Autodesk Inventor part; units mm, degrees
ref_plane "YZ Plane" through (0, 0, 0) normal (1, 0, 0) x (0, 1, 0)
ref_plane "XZ Plane" through (0, 0, 0) normal (0, 1, 0) x (-1, 0, 0)
ref_plane "XY Plane" through (0, 0, 0) normal (0, 0, 1) x (1, 0, 0)
sketch "Sketch1" plane through (0, 0, 0) normal (0, 0, 1) x (1, 0, 0)
  line L0 (-12.5, 71.5) -> (12.5, 71.5)
  line L1 (12.5, 71.5) -> (12.5, 0)
  line L2 (12.5, 0) -> (-12.5, 0)
  line L3 (-12.5, 0) -> (-12.5, 71.5)
  line L4 (-49.5, 71.5) -> (12.5, 71.5)
  line L5 (12.5, 71.5) -> (12.5, 38)
  line L6 (12.5, 38) -> (-49.5, 38)
  line L7 (-49.5, 38) -> (-49.5, 71.5)
  point P0 (0, 0)
  point P1 (0, 0)
  dimension "d0" = 25
  dimension "d1" = 71.5
  dimension "d2" = 62
  dimension "d3" = 33.5
extrude "Plate1" add sketch "Sketch1" along normal blind 2.5
sketch "Sketch2" plane through (12.5, 2.5, 0) normal (0, -1, 0) x (1, 0, 0)
  line L0 (-25, 0) -> (0, 0)
  line L1 (0, 0) -> (0, 27.5)
  line L2 (0, 27.5) -> (-25, 27.5)
  line L3 (-25, 27.5) -> (-25, 0)
edge flange "Flange1" height 27.5 angle 90 thickness 2.5 bend radius 2.5 thickness toward (0, -1, 0) relief tear relief width 2.5 relief depth 1.25 edges at (0, 0, 2.5) wall of the first edge with corners at (-12.5, 2.5, 0) (12.5, 2.5, 0) (12.5, 2.5, 27.5) (-12.5, 2.5, 27.5)
bend "Bend1"
corner "Corner1"
fillet "Fillet1" radius 12.5 1 edges at (-12.5, 1.25, 27.5)
fillet "Fillet2" radius 12.5 1 edges at (12.5, 1.25, 27.5)
sketch "Sketch5" plane through (-12.5, 0, 5) normal (0, -1, 0) x (1, 0, 0)
  line L0 (9.5, 14.3) -> (15.5, 14.3)
  line L1 (15.5, 14.3) -> (15.5, 5.7)
  line L2 (15.5, 5.7) -> (9.5, 5.7)
  line L3 (9.5, 5.7) -> (9.5, 14.3)
  arc A0 (25, 10) -> (0, 10) centre (12.5, 10) ccw
  arc A1 (9.5, 14.3) -> (9.5, 5.7) centre (12.5, 10) ccw
  arc A2 (15.5, 5.7) -> (15.5, 14.3) centre (12.5, 10) ccw
  line L4 (9.5, 5.7) -> (9.5, 14.3)
  line L5 (15.5, 5.7) -> (15.5, 14.3)
  point P0 (12.5, -5)
  point P1 (12.5, 14.3)
  point P2 (12.5, 22.5)
  dimension "d20" = 8.6
  dimension "d21" = 6
extrude "Cut1" cut sketch "Sketch5" against normal blind 2.5
sketch "Sketch6" plane through (0, 0, 2.5) normal (0, 0, 1) x (1, 0, 0)
  line L0 (12.5, 71.5) -> (-49.5, 71.5)
  line L1 (12.5, 71.5) -> (-13.5, 71.5)
  line L2 (-13.5, 71.5) -> (-13.5, 65)
  line L3 (-13.5, 65) -> (12.5, 65)
  line L4 (12.5, 65) -> (12.5, 71.5)
  line L5 (-3, 65) -> (12.5, 65)
  line L6 (12.5, 65) -> (12.5, 49.5)
  line L7 (12.5, 49.5) -> (-3, 65)
  point P0 (0, 0)
  dimension "d24" = 26
  dimension "d25" = 6.5
  dimension "d26" = 15.5
  dimension "d27" = 15.5
extrude "Cut2" cut sketch "Sketch6" against normal blind 2.5
fillet "Fillet3" radius 0.5 1 edges at (-13.5, 65, 1.25)
fillet "Fillet4" radius 8 2 edges at (-3, 65, 1.25) (12.5, 49.5, 1.25)
sketch "Sketch7" plane through (0, 0, 2.5) normal (0, 0, 1) x (1, 0, 0)
  line L0 (-12.5, 38) -> (-49.5, 38)
  line L1 (-12.5, 38) -> (-18.5, 38)
  line L2 (-12.5, 38) -> (-12.5, 32)
  line L3 (-12.5, 5) -> (-12.5, 38)
  line L4 (-12.5, 32) -> (-18.5, 38)
  point P0 (0, 0)
  dimension "d32" = 6
  dimension "d33" = 6
sheet face with bend "Face2" sketch "Sketch7" thickness 2.5 toward (0, 0, -1) bend radius 2.5
bend "Bend2"
sketch "Sketch8" plane through (0, 0, 2.5) normal (0, 0, 1) x (1, 0, 0)
  line L0 (-49.5, 71.5) -> (-49.5, 38)
  line L1 (-49.5, 38) -> (-36, 38)
  line L2 (-18.5, 38) -> (-49.5, 38)
  line L3 (-49.5, 38) -> (-49.5, 54.5)
  line L4 (-49.5, 54.5) -> (-43, 54.5)
  line L5 (-49.5, 54.5) -> (-49.5, 47.5)
  line L6 (-49.5, 54.5) -> (-42.5, 47.5)
  line L7 (-36, 38) -> (-42.5, 38)
  line L8 (-36, 38) -> (-36, 45)
  line L9 (-36, 38) -> (-42.5, 45)
  line L10 (-42.5, 45) -> (-42.5, 47.5)
  point P0 (0, 0)
  dimension "d39" = 13.5
  dimension "d40" = 16.5
  dimension "d41" = 6.5
  dimension "d42" = 7
  dimension "d43" = 6.5
  dimension "d44" = 7
extrude "Cut3" cut sketch "Sketch8" against normal blind 2.5
fillet "Fillet5" radius 1 1 edges at (-42.5, 47.5, 1.25)
sketch "Sketch9" plane through (0, 0, 2.5) normal (0, 0, 1) x (1, 0, 0)
  line L0 (-49.5, 71.5) -> (-13.5, 71.5)
  line L1 (-49.5, 54.5) -> (-49.5, 71.5)
  point P0 (0, 0)
  point P1 (-31.5, 49)
  dimension "d48" = 22.5
  dimension "d49" = 18
hole "Hole1" at (-31.5, 49, 2.5) direction (0, 0, -1) diameter 6 end through all
sketch "Sketch10" plane through (0, 0, 2.5) normal (0, 0, 1) x (1, 0, 0)
  line L0 (-46, 68.5) -> (-16.5, 68.5)
  line L1 (-16.5, 68.5) -> (-16.5, 59)
  line L2 (-16.5, 59) -> (-46, 59)
  line L3 (-46, 59) -> (-46, 68.5)
  line L4 (-49.5, 54.5) -> (-49.5, 71.5)
  line L5 (-16.5, 59) -> (-27.5, 59)
  line L6 (-16.5, 59) -> (-16.5, 52)
  circle A0 centre (-19, 52) radius 2.5
  line L7 (-49.5, 71.5) -> (-13.5, 71.5)
  line L8 (-21.4366, 52.5597) -> (-27.5, 59)
  point P0 (0, 0)
  dimension "d57" = 29.5
  dimension "d58" = 9.5
  dimension "d59" = 3.5
  dimension "d60" = 3
  dimension "d61" = 11
  dimension "d63" = 5
  dimension "d64" = 19.5
  dimension "d65" = 30.5
extrude "Cut4" cut sketch "Sketch10" against normal blind 2.5
equation "\"d22\" = Thickness"
equation "\"d28\" = Thickness"
equation "\"d45\" = Thickness"
equation "\"d55\" = Thickness"
equation "\"d66\" = Thickness"
equation "\"d68\" = Thickness"
equation "\"d5\" = BendReliefWidth"
equation "\"d6\" = BendReliefDepth"
equation "\"d7\" = MinimumRemnant"
equation "\"d8\" = BendRadius"
equation "\"d11\" = BendRadius"
equation "\"d12\" = CornerReliefSize"
equation "\"d13\" = GapSize"
equation "\"d14\" = JacobiRadiusSize"
equation "\"d34\" = BendRadius"
equation "\"d35\" = BendReliefWidth"
equation "\"d37\" = MinimumRemnant"
equation "\"d36\" = BendReliefDepth"
equation "\"d38\" = BendRadius"
equation "\"BendRadius\" = Thickness"
equation "\"BendReliefWidth\" = Thickness"
equation "\"BendReliefDepth\" = 0.5 * Thickness"
equation "\"MinimumRemnant\" = 2 * Thickness"
equation "\"TransitionRadius\" = BendRadius"
equation "\"JacobiRadiusSize\" = BendRadius"
equation "\"GapSize\" = Thickness"
equation "\"d4\" = BendRadius"
properties part number "Luxcan P2"
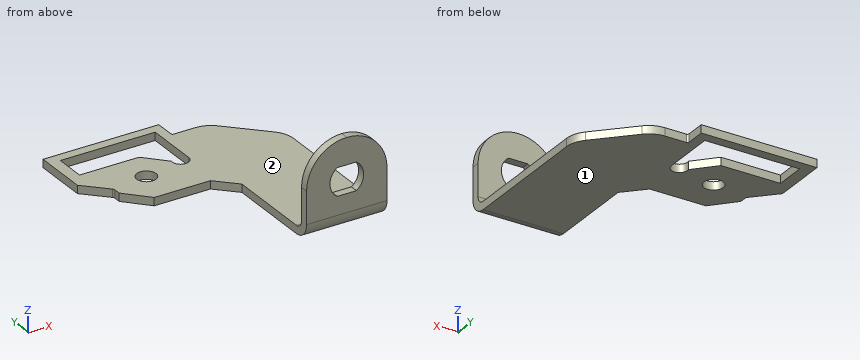
CAD build for the part. Positions are in the model's coordinates, mm. Face numbers are marked on the shaded views. A direction names the side the tool comes from. Give positions to 0.01 mm unless a question says otherwise; leave off trailing zeros. Loops run counter-clockwise (first coordinate to the right, second up) from the corner with the lowest first, then second, coordinate; pieces in that order, holes last. Notation, with made-up numbers: M 50.5,85.5 L 58.5,85.5 A26 cw 58.5,109.5 Z; hole C -20,34 d5. An arc over 180 degrees is marked long. One line per question, with ' | ' between items. Start each with the question number.
1. Saw through at A-A on y = 61.5. Give the cut face in (x, z).
2. 3-axis set-ups, long thin cutter, end or side, ignore diameter. For the marked faces 1 and 2: which of +Z, -Z, +X, -X, +Y, -Y reach the whole face in a straight line?
3. Saw through at B-B on x = -31.5. Give the cut face in (y, z).
4. Saw through at D-D on y = 11. Give the cut face in (x, z).
5. Saw through at C-C on z = 12.25. Give the cut face in (x, y).
6. Flat gauge pins, fed straight in: pin 1 (2 mm diameter, centred on x = 0.5, y = 1.5, fed in from -Z); pin 2 (2 mm diameter, centred on x = -10.5, z = 1.5, fed in from +Y); pin 3 (5 mm diameter, centred on x = -26, y = 35, fed in from -Z); pin 4 (1.2 mm diameter, centred on x = -27.5, z = 1.5, fed in from -Y). Where does each tip first touch, or does it go through?
7. Probe L1, parallel to Y at x = -31.5, z = 1.5; L2, parallel to Y at x = -19, z = 1.4; L3, parallel to Z at x = 2.5, y = 19. List the from-to ranges inside material, lowest first. Write a range as from..to.
Result sheet:
1) outline: M -49.5,0 L -46,0 L -46,2.5 L -49.5,2.5 Z; M -16.5,0 L 0.5,0 L 0.5,2.5 L -16.5,2.5 Z
2) face 1: -Z, +X, -X, +Y, -Y | face 2: +Z, +X, -X, +Y
3) outline: M 38,0 L 46,0 L 46,2.5 L 38,2.5 Z; M 52,0 L 59,0 L 59,2.5 L 52,2.5 Z; M 68.5,0 L 71.5,0 L 71.5,2.5 L 68.5,2.5 Z
4) outline: M -12.5,0 L 12.5,0 L 12.5,2.5 L -12.5,2.5 Z
5) outline: M -12.5,0 L -4.46,0 L -4.46,2.5 L -12.5,2.5 Z; M 4.46,0 L 12.5,0 L 12.5,2.5 L 4.46,2.5 Z
6) pin 1: stops at z = 0.67 | pin 2: stops at y = 65 | pin 3: passes through | pin 4: stops at y = 38
7) L1: y = 38..46, 52..59, 68.5..71.5 | L2: y = 38..49.5, 68.5..71.5 | L3: z = 0..2.5
